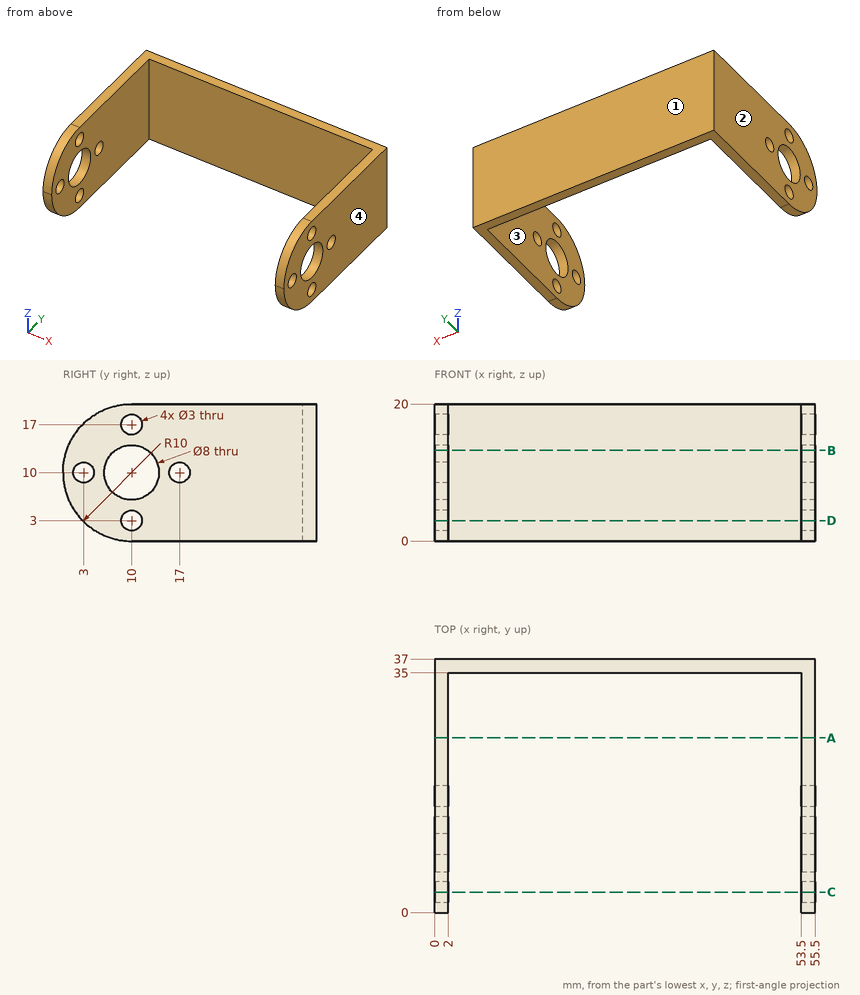
Design review of the part shown in the three views and the two pictorial views. Dimensions are in mm from the part's minimum x, y and z. Coordinates: 2 decimals unless noted, no trailing zeros. Loops run counter-clockwise (first coordinate to the right, second up) from the corner with the lowest first, then second, coordinate; pieces in that order, holes last. Notation, with made-up numbers: (8.25, 53) -> (66.25, 53) arc R30 ccw to (66.25, 83) -> close; hole circle Ø1 at (22, 25). An arc over 180 degrees is marked (long way). Answer as CSV lines item,"result".
Item 1: Take a section at A-A, the plane y = 25.5. State the section outline as (x, z) points.
Results below:
outline,"(0, 0) -> (2, 0) -> (2, 20) -> (0, 20) -> close; (53.5, 0) -> (55.5, 0) -> (55.5, 20) -> (53.5, 20) -> close"
Item 2: Draft analysis for pull direction X (two halves, no side actions). For the marked faces 1, 2, 3 and 4, state which applies: +X half, -X half, draft (parallel to the pull), parting line (faces both ways), or undercut.
Results below:
face 1,"draft"
face 2,"-X half"
face 3,"undercut"
face 4,"+X half"
Item 3: Take a section at B-B, the plane z = 13.25. State the section outline as (x, y) points, and give its area (3 significant figures).
Results below:
outline,"(0, 0.54) -> (2, 0.54) -> (2, 7.67) -> (0, 7.67) -> close; (0, 12.33) -> (2, 12.33) -> (2, 35) -> (53.5, 35) -> (53.5, 12.33) -> (55.5, 12.33) -> (55.5, 37) -> (0, 37) -> close; (53.5, 0.54) -> (55.5, 0.54) -> (55.5, 7.67) -> (53.5, 7.67) -> close"
area,"230 mm2"
Item 4: Insertion check: pin 1 (6 mm diameter, centred on x = 17.5, z = 7, fed in from -Y). The pin has a flat end and moves straight along its axis. Give the tip position at first contact, or say it passes through.
Results below:
pin 1,"stops at y = 35"
Item 5: Take a section at C-C, the plane y = 3. State the section outline as (x, z) points, and give its area (3 significant figures).
Results below:
outline,"(0, 2.86) -> (2, 2.86) -> (2, 8.5) -> (0, 8.5) -> close; (0, 11.5) -> (2, 11.5) -> (2, 17.14) -> (0, 17.14) -> close; (53.5, 2.86) -> (55.5, 2.86) -> (55.5, 8.5) -> (53.5, 8.5) -> close; (53.5, 11.5) -> (55.5, 11.5) -> (55.5, 17.14) -> (53.5, 17.14) -> close"
area,"45.1 mm2"
Item 6: Take a section at D-D, the plane z = 3. State the section outline as (x, y) points.
Results below:
outline,"(0, 2.86) -> (2, 2.86) -> (2, 8.5) -> (0, 8.5) -> close; (0, 11.5) -> (2, 11.5) -> (2, 35) -> (53.5, 35) -> (53.5, 11.5) -> (55.5, 11.5) -> (55.5, 37) -> (0, 37) -> close; (53.5, 2.86) -> (55.5, 2.86) -> (55.5, 8.5) -> (53.5, 8.5) -> close"
Item 7: For L1, parallel to Z at x = 54, y = 10; L2, parallel to X at y = 4.5, z = 16.25; L3, parallel to Z at x = 1, y = 17, list the stretches that pass through material, from the lowest coordinate up.
Results below:
L1,"z = 0 to 1.5, 4.5 to 6, 14 to 15.5, 18.5 to 20"
L2,"x = 0 to 2, 53.5 to 55.5"
L3,"z = 0 to 8.5, 11.5 to 20"
